from build123d import *

# Parameters (mm, degrees)
SKETCH1_R           = 1
BOSS_EXTRUDE1_DEPTH = 12.7


with BuildPart() as part:
    # Sketch1 → Boss-Extrude1 (new body)
    # profile 1 of 6: a face of its own
    with BuildSketch(Plane(origin=(0, 0, 0), x_dir=(1, 0, 0), z_dir=(0, 1, 0))):
        with BuildLine():
            Line((35.3, 48), (0, 48))
            ThreePointArc((0, 48), (19.271411924, 43.961490903), (35.3, 32.525528435))
            Line((35.3, 32.525528435), (35.3, 48))
        make_face()
    # profile 2 of 6: a face of its own
    with BuildSketch(Plane(origin=(0, 0, 0), x_dir=(1, 0, 0), z_dir=(0, 1, 0))):
        with BuildLine():
            Line((48, 32.525528435), (35.3, 32.525528435))
            ThreePointArc((35.3, 32.525528435), (44.712414383, 17.458522274), (48, 0))
            Line((48, 0), (48, 32.525528435))
        make_face()
    # profile 3 of 6: a face of its own
    with BuildSketch(Plane(origin=(0, 0, 0), x_dir=(1, 0, 0), z_dir=(0, 1, 0))):
        with BuildLine():
            ThreePointArc((-35.3, 32.525528435), (-19.271411924, 43.961490903), (0, 48))
            Line((0, 48), (-35.3, 48))
            Line((-35.3, 48), (-35.3, 32.525528435))
        make_face()
    # profile 4 of 6: a face of its own
    with BuildSketch(Plane(origin=(0, 0, 0), x_dir=(1, 0, 0), z_dir=(0, 1, 0))):
        with BuildLine():
            ThreePointArc((-48, 0), (-44.712414383, 17.458522274), (-35.3, 32.525528435))
            Line((-35.3, 32.525528435), (-48, 32.525528435))
            Line((-48, 32.525528435), (-48, 0))
        make_face()
    # profile 5 of 6: a face of its own
    with BuildSketch(Plane(origin=(0, 0, 0), x_dir=(1, 0, 0), z_dir=(0, 1, 0))):
        with BuildLine():
            ThreePointArc((35.3, 32.525528435), (19.271411924, 43.961490903), (0, 48))
            ThreePointArc((0, 48), (-19.271411924, 43.961490903), (-35.3, 32.525528435))
            ThreePointArc((-35.3, 32.525528435), (-44.712414383, 17.458522274), (-48, 0))
            Line((-48, 0), (-40, 0))
            ThreePointArc((-40, 0), (0, 40), (40, 0))
            Line((40, 0), (48, 0))
            ThreePointArc((48, 0), (44.712414383, 17.458522274), (35.3, 32.525528435))
        make_face()
        with Locations(Location((-34.400585229, 27.433551282, 0), (0, 0, 270))):
            Circle(SKETCH1_R, mode=Mode.SUBTRACT)
        with Locations(Location((0, 44, 0), (0, 0, 270))):
            Circle(SKETCH1_R, mode=Mode.SUBTRACT)
        with Locations(Location((34.400585229, 27.433551282, 0), (0, 0, 270))):
            Circle(SKETCH1_R, mode=Mode.SUBTRACT)
    # profile 6 of 6: a face of its own
    with BuildSketch(Plane(origin=(0, 0, 0), x_dir=(1, 0, 0), z_dir=(0, 1, 0))):
        with BuildLine():
            ThreePointArc((-48, 0), (0, -48), (48, 0))
            Line((48, 0), (40, 0))
            ThreePointArc((40, 0), (0, -40), (-40, 0))
            Line((-40, 0), (-48, 0))
        make_face()
        with Locations(Location((-19.090884521, -39.642630188, 0), (0, 0, 270))):
            Circle(SKETCH1_R, mode=Mode.SUBTRACT)
        with Locations(Location((-42.896828136, -9.790921094, 0), (0, 0, 270))):
            Circle(SKETCH1_R, mode=Mode.SUBTRACT)
        with Locations(Location((19.090884521, -39.642630188, 0), (0, 0, 270))):
            Circle(SKETCH1_R, mode=Mode.SUBTRACT)
        with Locations(Location((42.896828136, -9.790921094, 0), (0, 0, 270))):
            Circle(SKETCH1_R, mode=Mode.SUBTRACT)
    extrude(amount=BOSS_EXTRUDE1_DEPTH)


solid = part.part
Check sheet for the modelled part. Datum: model origin and axes. Units: mm. A direction names the side the tool comes from. Give positions to 0.01 mm unless a question says otherwise; leave off trailing zeros. Write each loop counter-clockwise with the first axis right and the second up, starting at its lowest first coordinate (ties: lowest second). Pieces come first, ordered by that corner, then holes. Notation, with made-up numbers: (13.25, 18) -> (18.25, 18) arc R32 ccw to (18.25, 53) -> close; hole circle Ø1 at (-4, 24). An arc over 180 degrees is marked (long way). One line per item, written item: value. Start each with the question number.
Item 1: Gauge pin test, flat ends, axial feed: pin 1 (1.6 mm diameter, centred on x = -42.9, z = 9.79, fed in from -Y); pin 2 (3 mm diameter, centred on y = 10.5, z = 4, fed in from +X); pin 3 (4 mm diameter, centred on y = 5.5, z = -41, fed in from +X); pin 4 (1 mm diameter, centred on y = 5, z = 37.5, fed in from -X). Record the tip position at first contact, or that the pin passes through.
Item 2: Section check C-C on y = 7.25. State how many separate pieces and enclosed holes the cut face has, then the cut area to 3 significant figures.
Item 3: Section check B-B on z = -24. Record the cut outline in (x, y), then the cut area to 3 significant figures.
Item 4: Section check A-A on x = 16.5. Record the cut outline in (y, z), then the cut area to 3 significant figures.
Item 5: Draft check along Z on faces 4 (the flat face through (48, 6, -16)), 5 (the cylindrical face through (-32, 6, -24)), 6 (the flat face through (-42, 6, -32.526)). Enter one of: +Z half, -Z half, draft (parallel to the pull), parting line (faces both ways), or undercut.
Item 6: Tool access check on faces 1 (the flat face through (-35.3, 6, -40)), 2 (the cylindrical face through (-1.06, 6.26, 47.99)), 3 (the flat face through (35.3, 6, -40)). Record the directions out of +Z, -Z, +X, -X, +Y, -Y that give a thin tool (end or side, any length) a straight path to the whole face; none if there is none.
Item 7: Material ranges on probe 1 along X at (y, z) = (2, -0.5); probe 2 along X at (y, z) = (11.5, -14.5); probe 3 along Z at (x, y) = (23, 9.75), recorded low to high. Write a range as from..to.
Results list:
1. pin 1: through
1. pin 2: x = 47.93
1. pin 3: x = 35.3
1. pin 4: x = -30.58
2. separate pieces: 1
2. enclosed holes: 8
2. area: 2,790 mm²
3. outline: (-48, 0) -> (-32, 0) -> (-32, 12.7) -> (-48, 12.7) -> close; (32, 0) -> (48, 0) -> (48, 12.7) -> (32, 12.7) -> close
3. area: 406 mm²
4. outline: (0, -48) -> (12.7, -48) -> (12.7, -36.44) -> (0, -36.44) -> close; (0, 36.44) -> (12.7, 36.44) -> (12.7, 45.07) -> (0, 45.07) -> close
4. area: 257 mm²
5. face 4: draft
5. face 5: undercut
5. face 6: -Z half
6. face 1: -Z, -X, +Y, -Y
6. face 2: +Z, +Y, -Y
6. face 3: -Z, +X, +Y, -Y
7. probe 1: -48..-40, 40..48
7. probe 2: -48..-37.28, 37.28..48
7. probe 3: -48..-32.73, 32.73..42.13
